from build123d import *

# Parameters (mm, degrees)
SKETCH1_W           = 100
SKETCH1_H           = 100
BOSS_EXTRUDE1_DEPTH = 155
SKETCH2_W           = 60
SKETCH2_H           = 100
CUT_EXTRUDE1_DEPTH  = 20
SKETCH3_R           = 3.75
CUT_EXTRUDE2_DEPTH  = 4
SKETCH4_R           = 2.5
CUT_EXTRUDE3_DEPTH  = 192.115148536
SKETCH6_R           = 3.75
CUT_EXTRUDE5_DEPTH  = 4
SKETCH9_R           = 2.5
CUT_EXTRUDE7_DEPTH  = 50


with BuildPart() as part:
    # Sketch1 → Boss-Extrude1 (new body)
    with BuildSketch(Plane(origin=(0, 0, 0), x_dir=(1, 0, 0), z_dir=(0, 1, 0))):
        Rectangle(SKETCH1_W, SKETCH1_H)
    extrude(amount=BOSS_EXTRUDE1_DEPTH)

    # Sketch2 → Cut-Extrude1 (cut)
    with BuildSketch(Plane.ZY.offset(50)):
        with Locations((0, 77.5)):
            Rectangle(SKETCH2_W, SKETCH2_H)
    cut_extrude1 = extrude(amount=-CUT_EXTRUDE1_DEPTH, mode=Mode.SUBTRACT)

    # Mirror1: Cut-Extrude1 across plane
    add(cut_extrude1.mirror(Plane(origin=(0, 0, 0), x_dir=(0, 0, 1), z_dir=(1, 0, 0))), mode=Mode.SUBTRACT)

    # Sketch3 → Cut-Extrude2 (cut)
    with BuildSketch(Plane.XY.offset(50)):
        with Locations((-40, 100)):
            Circle(SKETCH3_R)
        with Locations(Location((-40, 55, 0), (0, 0, 180))):
            Circle(SKETCH3_R)
        with Locations((40, 55)):
            Circle(SKETCH3_R)
        with Locations(Location((40, 100, 0), (0, 0, 180))):
            Circle(SKETCH3_R)
    cut_extrude2 = extrude(amount=-CUT_EXTRUDE2_DEPTH, mode=Mode.SUBTRACT)

    # Mirror2: Cut-Extrude2 across plane
    add(cut_extrude2.mirror(Plane.XY), mode=Mode.SUBTRACT)

    # Sketch4 → Cut-Extrude3 (cut, through all)
    with BuildSketch(Plane.XY.offset(50)):
        with Locations(Location((-40, 100, 0), (0, 0, 180))):
            Circle(SKETCH4_R)
        with Locations((40, 100)):
            Circle(SKETCH4_R)
        with Locations((40, 55)):
            Circle(SKETCH4_R)
        with Locations((-40, 55)):
            Circle(SKETCH4_R)
    extrude(amount=-CUT_EXTRUDE3_DEPTH, mode=Mode.SUBTRACT)

    # Sketch6 → Cut-Extrude5 (cut)
    with BuildSketch(Plane.XZ):
        with Locations(Location((-40, 15, 0), (0, 0, 270))):
            Circle(SKETCH6_R)
        with Locations(Location((40, 15, 0), (0, 0, 90))):
            Circle(SKETCH6_R)
        with Locations(Location((40, -15, 0), (0, 0, 270))):
            Circle(SKETCH6_R)
        with Locations(Location((-40, -15, 0), (0, 0, 90))):
            Circle(SKETCH6_R)
    extrude(amount=-CUT_EXTRUDE5_DEPTH, mode=Mode.SUBTRACT)

    # Sketch9 → Cut-Extrude7 (cut)
    with BuildSketch(Plane.XZ):
        with Locations(Location((-40, 15, 0), (0, 0, 270))):
            Circle(SKETCH9_R)
        with Locations(Location((40, 15, 0), (0, 0, 90))):
            Circle(SKETCH9_R)
        with Locations(Location((40, -15, 0), (0, 0, 270))):
            Circle(SKETCH9_R)
        with Locations(Location((-40, -15, 0), (0, 0, 270))):
            Circle(SKETCH9_R)
    extrude(amount=-CUT_EXTRUDE7_DEPTH, mode=Mode.SUBTRACT)


solid = part.part
Read the model definition and answer for the solid it produces. Units are mm, in the model's axes. A direction names the side the tool comes from. Coordinates: 2 decimals unless noted, no trailing zeros. Write each loop counter-clockwise with the first axis right and the second up, starting at its lowest first coordinate (ties: lowest second). Pieces come first, ordered by that corner, then holes. Notation, with made-up numbers: (19, -38) -> (45, -38) arc R27 cw to (45, -15) -> close; hole circle Ø11 at (-15.75, 16). An arc over 180 degrees is marked (long way). Return JSON: item names as keys, results as strings.
(1) Consider line 1 along X through (y, z) = (3.25, -15); line 2 along Y through (x, z) = (-40, -48.4); line 3 along X through (y, z) = (21, -15). Determine where each line is inside the solid, lowest interval first. Write a range as from..to.
Answers below:
{"line 1": "-50..-43.75, -36.25..36.25, 43.75..50", "line 2": "0..51.25, 58.75..96.25, 103.75..155", "line 3": "-50..-42.5, -37.5..37.5, 42.5..50"}
(2) For a pull along Y with two mould halves and no side action, classify faces 1 (the flat face through (-37, 4, 15)), 2 (the flat face through (50, 76, 34)), 3 (the cylindrical face through (42.31, 54.04, 38.11)) as pulls with the +Y half, pulls with the -Y half, needs draft (parallel to the pull), parting line crosses it, or undercut.
Answers below:
{"face 1": "pulls with the -Y half", "face 2": "needs draft", "face 3": "undercut"}
(3) Each of these flat-tipped pins is pushed along its axis until it touches: P1, Ø1.5, axis at y = 125.5, z = -11.5, coming from the -X side; P2, Ø12, axis at y = 72, z = 22.5, coming from the +X side; P3, Ø6, axis at x = 41, z = -14.5, coming from the -Y side; P4, Ø6, axis at x = -40, z = -15, coming from the -Y side. Where does it stop, or does it pass through?
Answers below:
{"P1": "x = -30", "P2": "x = 30", "P3": "y = 0", "P4": "y = 4"}
(4) The part is cut by section C-C on x = 40. State how many separate pieces and enclosed holes the cut face has, then the cut area to 4 significant figures.
Answers below:
{"separate pieces": "6", "enclosed holes": "0", "area": "8,765 mm^2"}
(5) The part is cut by section A-A on z = -15. Give the vertices of the cut face in (x, y).
Answers below:
{"outline": "(-50, 0) -> (-43.75, 0) -> (-43.75, 4) -> (-42.5, 4) -> (-42.5, 27.5) -> (-50, 27.5) -> close; (-50, 127.5) -> (-30, 127.5) -> (-30, 27.5) -> (-37.5, 27.5) -> (-37.5, 4) -> (-36.25, 4) -> (-36.25, 0) -> (36.25, 0) -> (36.25, 4) -> (37.5, 4) -> (37.5, 27.5) -> (30, 27.5) -> (30, 127.5) -> (50, 127.5) -> (50, 155) -> (-50, 155) -> close; (42.5, 4) -> (43.75, 4) -> (43.75, 0) -> (50, 0) -> (50, 27.5) -> (42.5, 27.5) -> close"}
(6) Which of the six approach directions +Z, -Z, +X, -X, +Y, -Y give full straight-line access (tool end or side, diameter ignored) to faces 4 (the flat face through (-30, 78, 0)), 5 (the cylindrical face through (40.488, 96.282, 48.028)), 6 (the flat face through (-43, 100, -46))?
Answers below:
{"face 4": "-X", "face 5": "+Z", "face 6": "-Z"}
(7) The part is cut by section B-B on y = 67.5. Give the vertices of the cut face in (x, z), then the cut area to 3 significant figures.
Answers below:
{"outline": "(-50, -50) -> (50, -50) -> (50, -30) -> (30, -30) -> (30, 30) -> (50, 30) -> (50, 50) -> (-50, 50) -> (-50, 30) -> (-30, 30) -> (-30, -30) -> (-50, -30) -> close", "area": "7,600 mm^2"}
